Work out the finished part from the listing and answer in its coordinate system (mm). A direction names the side the tool comes from. Coordinates: 2 decimals unless noted, no trailing zeros. Order: outer loops, then holes, each group sorted by start corner. A loop starts at its lowest first (then second) coordinate and runs counter-clockwise, first axis right, second up.
1. The part is cut by section A-A, the plane x = -4. Give the vertices of the cut face in (y, z).
2. A tool of negligible diameter and unlimited length cuts with its end or side. For faces 4 (the cylindrical face through (-21.706, 24.591, 21.232)), 5 (the flat face through (-25, -21, 10)), 6 (the cylindrical face through (-23.38, 21.557, 0.937)), from which of +Z, -Z, +X, -X, +Y, -Y can it reach the whole face along a straight path? Write none if from no direction.
3. The part is cut by section C-C, the plane x = -16.5. Give the vertices of the cut face in (y, z).
4. Determine the mould class of faces 1 (the flat face through (0, -27.8, 10)), 2 (the cylindrical face through (-22.13, -22.28, 0.94)), 3 (the flat face through (-24, 24, 22.7)) for opening direction Y: +Y half, -Y half, draft (parallel to the pull), parting line (faces both ways), or undercut.
5. Flat-ended cylindrical pins translate along their axes: pin 1 Ø0.8 at (x, y) = (-3, 27) entering from +Z; pin 2 Ø2.5 at (x, y) = (24.5, 24.5) entering from -Z. Find the tip coordinate at first contact, or state that the pin passes through.
6. Find the intervals of material crossed by probe 1 along Y at (x, z) = (-23.9, 1.35); probe 2 along X at (y, z) = (-10, 7.5), in increasing order.
7. The part is cut by section B-B, the plane z = 19.25. Give the vertices of the cut face in (x, y), then the cut area to 3 significant figures.
```python
from build123d import *

# Parameters (mm, degrees)
SKICA1_W                 = 5.8
SKICA1_H                 = 5.8
SKICA1_W_2               = 1
SKICA1_H_2               = 42
SKICA1_W_3               = 42
SKICA1_H_3               = 1
P_IDAT_VYSUNUT_M2_DEPTH  = 20
ZAOBLIT1_R               = 2.5
SKICA2_R                 = 2.4
ODEBRAT_VYSUNUT_M1_DEPTH = 1.9
SKICA3_R                 = 2.3
P_IDAT_VYSUNUT_M3_DEPTH  = 2.7
ZKOSEN_1_SIZE            = 0.2
SKICA4_W                 = 10.16
SKICA4_H                 = 5.08
ODEBRAT_VYSUNUT_M2_DEPTH = 68.7


with BuildPart() as part:
    # Skica1 → Přidat vysunutím2 (new body)
    with BuildSketch(Plane.XY):
        Polygon((-27.8, 27.8), (-27.8, 21), (-26.8, 21), (-26.8, 26.8), (-21, 26.8), (-21, 27.8), align=None)
        with Locations((-23.9, 23.9)):
            Rectangle(SKICA1_W, SKICA1_H)
        Polygon((26.8, 21), (27.8, 21), (27.8, 27.8), (21, 27.8), (21, 26.8), (26.8, 26.8), align=None)
        with Locations((23.9, 23.9)):
            Rectangle(SKICA1_W, SKICA1_H)
        Polygon((21, -26.8), (21, -27.8), (27.8, -27.8), (27.8, -21), (26.8, -21), (26.8, -26.8), align=None)
        with Locations((23.9, -23.9)):
            Rectangle(SKICA1_W, SKICA1_H)
        with Locations((-23.9, -23.9)):
            Rectangle(SKICA1_W, SKICA1_H)
        Polygon((-27.8, -27.8), (-21, -27.8), (-21, -26.8), (-26.8, -26.8), (-26.8, -21), (-27.8, -21), align=None)
        with Locations((-27.3, 0)):
            Rectangle(SKICA1_W_2, SKICA1_H_2)
        with Locations((0, -27.3)):
            Rectangle(SKICA1_W_3, SKICA1_H_3)
        with Locations((27.3, 0)):
            Rectangle(SKICA1_W_2, SKICA1_H_2)
        with Locations((0, 27.3)):
            Rectangle(SKICA1_W_3, SKICA1_H_3)
    extrude(amount=P_IDAT_VYSUNUT_M2_DEPTH)

    # Zaoblit1
    zaoblit1_edges = [part.edges().sort_by_distance(p)[0] for p in [
        (21, -21, 10),
        (21, 21, 10),
        (-21, 21, 10),
        (-21, -21, 10),
    ]]
    fillet(zaoblit1_edges, radius=ZAOBLIT1_R)

    # Skica2 → Odebrat vysunutím1 (cut)
    with BuildSketch(Plane(origin=(0, 0, 0), x_dir=(-1, 0, 0), z_dir=(0, 0, -1))):
        with Locations((-23.9, 23.9)):
            Circle(SKICA2_R)
        with Locations((23.9, 23.9)):
            Circle(SKICA2_R)
        with Locations((23.9, -23.9)):
            Circle(SKICA2_R)
        with Locations((-23.9, -23.9)):
            Circle(SKICA2_R)
    extrude(amount=-ODEBRAT_VYSUNUT_M1_DEPTH, mode=Mode.SUBTRACT)

    # Skica3 → Přidat vysunutím3 (add)
    with BuildSketch(Plane.XY.offset(20)):
        with Locations((-23.9, 23.9)):
            Circle(SKICA3_R)
        with Locations((23.9, 23.9)):
            Circle(SKICA3_R)
        with Locations((23.9, -23.9)):
            Circle(SKICA3_R)
        with Locations((-23.9, -23.9)):
            Circle(SKICA3_R)
    extrude(amount=P_IDAT_VYSUNUT_M3_DEPTH)

    # Zkosení1
    zkosen_1_edges = [part.edges().sort_by_distance(p)[0] for p in [
        (-26.2, 23.9, 22.7),
        (21.6, 23.9, 22.7),
        (21.6, -23.9, 22.7),
        (-26.2, -23.9, 22.7),
    ]]
    chamfer(zkosen_1_edges, length=ZKOSEN_1_SIZE)

    # Skica4 → Odebrat vysunutím2 (cut)
    with BuildSketch(Plane(origin=(0, -27.8, 0), x_dir=(-1, 0, 0), z_dir=(0, -1, 0))):
        with Locations((0.5, -4.54)):
            Rectangle(SKICA4_W, SKICA4_H)
    extrude(amount=-ODEBRAT_VYSUNUT_M2_DEPTH, mode=Mode.SUBTRACT)


solid = part.part
```
Geometry says:
1. outline: (-27.8, 0) - (-26.8, 0) - (-26.8, 2) - (-27.8, 2) - close; (-27.8, 7.08) - (-26.8, 7.08) - (-26.8, 20) - (-27.8, 20) - close; (26.8, 0) - (27.8, 0) - (27.8, 2) - (26.8, 2) - close; (26.8, 7.08) - (27.8, 7.08) - (27.8, 20) - (26.8, 20) - close
2. face 4: +Z
2. face 5: +Z, -Z
2. face 6: -Z
3. outline: (-27.8, 0) - (-26.8, 0) - (-26.8, 20) - (-27.8, 20) - close; (26.8, 0) - (27.8, 0) - (27.8, 20) - (26.8, 20) - close
4. face 1: -Y half
4. face 2: undercut
4. face 3: draft
5. pin 1: stops at z = 20
5. pin 2: stops at z = 1.9
6. probe 1: y = -27.8 to -26.3, -21.5 to -21, 21 to 21.5, 26.3 to 27.8
6. probe 2: x = -27.8 to -26.8, 26.8 to 27.8
7. outline: (-27.8, -27.8) - (27.8, -27.8) - (27.8, 27.8) - (-27.8, 27.8) - close; hole (-26.8, -21) - (-23.5, -21) arc R2.5 cw to (-21, -23.5) - (-21, -26.8) - (21, -26.8) - (21, -23.5) arc R2.5 cw to (23.5, -21) - (26.8, -21) - (26.8, 21) - (23.5, 21) arc R2.5 cw to (21, 23.5) - (21, 26.8) - (-21, 26.8) - (-21, 23.5) arc R2.5 cw to (-23.5, 21) - (-26.8, 21) - close
7. area: 348 mm2
